from build123d import *

# Parameters (mm, degrees)
F0_R          = 4.5
F1_DEPTH      = 65
F2_W          = 24.1539999843
F2_H          = 28
F2_W_2        = 25
F2_W_3        = 30
F2_H_2        = 80
F3_DEPTH      = 45.001
F4_R          = 4.5
F5_DEPTH      = 45.001
F6_R          = 4.5
F7_DEPTH      = 6.5
F8_R          = 4.5
F9_DEPTH      = 14.5
F10_T4_DEPTH  = 132.8518303197
F10_S5_R      = 17.5
F10_T6_DEPTH  = 68
F10_T10_DEPTH = 132.8518303197
F10_S11_R     = 17.5
F10_T12_DEPTH = 68
F11_R         = 2


# Not quite as in the source:
# - a fillet or chamfer that OpenCascade refuses, or shapes differently, is made with other operations: its cross-section is extruded or revolved along the edge and cut away or added
# - a pattern or mirror of a feature is missing from the dataset's text; its kind, count and spacing are read off the source's solid


with BuildPart() as f1:
    # F0 (on Front) → F1 (new body, symmetric)
    with BuildSketch(Plane.XZ):
        with BuildLine():
            Line((80, 17.5), (0, 17.5))
            ThreePointArc((0, 17.5), (-17.2437155554, 2.9840029898), (-5.880605574, -16.4823687036))
            Line((-5.880605574, -16.4823687036), (25, -27.5))
            Line((25, -27.5), (55, -27.5))
            Line((55, -27.5), (85.880605574, -16.4823687036))
            ThreePointArc((85.880605574, -16.4823687036), (97.2437155554, 2.9840029898), (80, 17.5))
        make_face()
        Circle(F0_R, mode=Mode.SUBTRACT)
        with Locations((80, 0)):
            Circle(F0_R, mode=Mode.SUBTRACT)
    extrude(amount=F1_DEPTH, both=True)

    # F2 (on face) → F3 (cut, through all)
    with BuildSketch(Plane.XY.offset(17.5)):
        with Locations((-12.0769999921, 51)):
            Rectangle(F2_W, F2_H)
        with Locations((12.5, 51)):
            Rectangle(F2_W_2, F2_H)
        with Locations((-12.0769999921, -51)):
            Rectangle(F2_W, F2_H)
        with Locations((12.5, -51)):
            Rectangle(F2_W_2, F2_H)
        Polygon((55, 40), (55, 0), (55, -40), (80, -40), (80, 40), align=None)
        with Locations((95, 0)):
            Rectangle(F2_W_3, F2_H_2)
    extrude(amount=-F3_DEPTH, mode=Mode.SUBTRACT)

    # F4 (on face) → F5 (cut, through all)
    with BuildSketch(Plane(origin=(0, 0, -27.5), x_dir=(1, 0, 0), z_dir=(0, 0, -1))):
        with Locations((40, 50)):
            Circle(F4_R)
        with Locations((40, -50)):
            Circle(F4_R)
    extrude(amount=-F5_DEPTH, mode=Mode.SUBTRACT)

    # F6 (on face) → F7 (cut)
    with BuildSketch(Plane.XY.offset(17.5)):
        Polygon((35.9585481157, 43), (44.0414518843, 43), (48.0829037687, 50), (44.0414518843, 57), (35.9585481157, 57), (31.9170962313, 50), align=None)
        with Locations((40, 50)):
            Circle(F6_R, mode=Mode.SUBTRACT)
        Polygon((44.0414518843, -57), (48.0829037687, -50), (44.0414518843, -43), (35.9585481157, -43), (31.9170962313, -50), (35.9585481157, -57), align=None)
        with Locations((40, -50)):
            Circle(F6_R, mode=Mode.SUBTRACT)
    extrude(amount=-F7_DEPTH, mode=Mode.SUBTRACT)

    # F8 (on face) → F9 (join)
    with BuildSketch(Plane.XZ.offset(65)):
        with BuildLine():
            ThreePointArc((85.880605574, -16.4823687036), (94.3031569513, -10.0831394529), (97.5, 0))
            ThreePointArc((97.5, 0), (92.3743686708, 12.3743686708), (80, 17.5))
            ThreePointArc((80, 17.5), (62.7562844446, -2.9840029898), (85.880605574, -16.4823687036))
        make_face()
        with Locations((80, 0)):
            Circle(F8_R, mode=Mode.SUBTRACT)
    f9 = extrude(amount=F9_DEPTH)

    # F9_copies: F9 across plane
    add(f9.mirror(Plane.ZX))

    # F10: chamfer of 5 x 15 on 2 edges, made by hand


with BuildPart() as f10_tool2:
    # F10_s3 → F10_t4 (new body)
    with BuildSketch(Plane.YZ.offset(118.9259151598)):
        Polygon((-60, 17.5), (-65, 2.5), (-65, 17.5), align=None)
    extrude(amount=-F10_T4_DEPTH)

    # F10_s5 → F10_t6 (cut, symmetric)
    with BuildSketch(Plane.XZ.offset(62.5)):
        with Locations((80, 0)):
            Circle(F10_S5_R)
    extrude(amount=F10_T6_DEPTH, both=True, mode=Mode.SUBTRACT)


with BuildPart() as f1_1:
    add(f1.part)

    # F10_t1: cut F10_tool2
    add(f10_tool2.part, mode=Mode.SUBTRACT)


with BuildPart() as f10_tool8:
    # F10_s9 → F10_t10 (new body)
    with BuildSketch(Plane.YZ.offset(118.9259151598)):
        Polygon((60, 17.5), (65, 2.5), (65, 17.5), align=None)
    extrude(amount=-F10_T10_DEPTH)

    # F10_s11 → F10_t12 (cut, symmetric)
    with BuildSketch(Plane.XZ.offset(-62.5)):
        with Locations((80, 0)):
            Circle(F10_S11_R)
    extrude(amount=F10_T12_DEPTH, both=True, mode=Mode.SUBTRACT)


with BuildPart() as f1_2:
    add(f1_1.part)

    # F10_t7: cut F10_tool8
    add(f10_tool8.part, mode=Mode.SUBTRACT)

    # F11
    f11_edges = [f1_2.edges().sort_by_distance(p)[0] for p in [
        (55, -40, -5),
        (55, 40, -5),
    ]]
    fillet(f11_edges, radius=F11_R)


solid = f1_2.part
The model under review builds one solid part; all positions refer to its coordinate system, in mm. A direction names the side the tool comes from. Coordinates: 2 decimals unless noted, no trailing zeros. Write each loop counter-clockwise with the first axis right and the second up, starting at its lowest first coordinate (ties: lowest second). Pieces come first, ordered by that corner, then holes. Notation, with made-up numbers: (28.25, 32) -> (73.25, 32) arc R28 ccw to (73.25, 51) -> close; hole circle Ø1 at (49, 43.5). An arc over 180 degrees is marked (long way). Answer in a Markdown table with one row per item.
1. We need section D-D, the plane z = -21.5. State the section outline as (x, y) points, and give its area (3 significant figures).
Answers below:
| item | result |
|---|---|
| outline | (8.18, -37) -> (25, -37) -> (25, -65) -> (71.82, -65) -> (71.82, -40) -> (57, -40) arc R2 cw to (55, -38) -> (55, 38) arc R2 cw to (57, 40) -> (71.82, 40) -> (71.82, 65) -> (25, 65) -> (25, 37) -> (8.18, 37) -> close; hole circle Ø9 at (40, -50); hole circle Ø9 at (40, 50) |
| area | 5,860 mm^2 |
2. For faces 1 (the flat face through (46.774, 62.465, 10.105)), 2 (the cylindrical face through (95.577, 63.862, 7.976)), 3 (the flat face through (46.034, 46.451, 14.296)), 4 (the flat face through (73, 40, 1)), 5 (the flat face through (9, -37, 0)), list the 3-axis set-ups (+Z, -Z, +X, -X, +Y, -Y) from which the entire face can be reached by the end or side of a thin tool; tool diameter is ignored.
Answers below:
| item | result |
|---|---|
| face 1 | +Z, -X, +Y |
| face 2 | +Y |
| face 3 | +Z |
| face 4 | +Z, -Z, +X |
| face 5 | +Z, -Z, -X, -Y |
3. Clearance check with flat-ended pins moving along their axes: pin 1 Ø12.5 at (x, z) = (-5, -2.5) entering from -Y; pin 2 Ø12 at (x, z) = (29.5, -5.5) entering from +Y; pin 3 Ø7 at (x, z) = (80, 0) entering from +Y; pin 4 Ø4 at (y, z) = (49.5, 4.5) entering from +X. State where each tip first meets the part, or that it passes through.
Answers below:
| item | result |
|---|---|
| pin 1 | stops at y = -37 |
| pin 2 | stops at y = 65 |
| pin 3 | passes through |
| pin 4 | stops at x = 97.32 |
4. We need section A-A, the plane x = 40. State the section outline as (y, z) points.
Answers below:
| item | result |
|---|---|
| outline | (-65, -27.5) -> (-54.5, -27.5) -> (-54.5, 11) -> (-57, 11) -> (-57, 17.5) -> (-60, 17.5) -> (-65, 2.5) -> close; (-45.5, -27.5) -> (45.5, -27.5) -> (45.5, 11) -> (43, 11) -> (43, 17.5) -> (-43, 17.5) -> (-43, 11) -> (-45.5, 11) -> close; (54.5, -27.5) -> (65, -27.5) -> (65, 2.5) -> (60, 17.5) -> (57, 17.5) -> (57, 11) -> (54.5, 11) -> close |
5. Draft analysis for pull direction Y (two halves, no side actions). For faces 6 (the flat face through (84, 79.5, -4)), 7 (the flat face through (40, -1, -27.5)), 8 (the flat face through (84, -79.5, -4)), 9 (the cylindrical face through (42.08, -46.01, -8.52)), state which applies: +Y half, -Y half, draft (parallel to the pull), parting line (faces both ways), or undercut.
Answers below:
| item | result |
|---|---|
| face 6 | +Y half |
| face 7 | draft |
| face 8 | -Y half |
| face 9 | undercut |
6. We need section C-C, the plane x = 88. State the section outline as (y, z) points, and give its area (3 significant figures).
Answers below:
| item | result |
|---|---|
| outline | (-79.5, -15.56) -> (-40, -15.56) -> (-40, 15.56) -> (-79.5, 15.56) -> close; (40, -15.56) -> (79.5, -15.56) -> (79.5, 15.56) -> (40, 15.56) -> close |
| area | 2,460 mm^2 |
7. We need section B-B, the plane z = -6.5. State the section outline as (x, y) points.
Answers below:
| item | result |
|---|---|
| outline | (-16.25, -37) -> (25, -37) -> (25, -65) -> (63.75, -65) -> (63.75, -79.5) -> (96.25, -79.5) -> (96.25, -40) -> (57, -40) arc R2 cw to (55, -38) -> (55, 38) arc R2 cw to (57, 40) -> (96.25, 40) -> (96.25, 79.5) -> (63.75, 79.5) -> (63.75, 65) -> (25, 65) -> (25, 37) -> (-16.25, 37) -> close; hole circle Ø9 at (40, -50); hole circle Ø9 at (40, 50) |
8. Wall thickness on probe 1 along Y at (x, z) = (40, -13.5); probe 2 along X at (y, z) = (50, 0.5); probe 3 along Y at (x, z) = (87, 15): over which ranges is each line inside the solid? List them lowest first. Write a range as [from, to].
Answers below:
| item | result |
|---|---|
| probe 1 | y = [-65, -54.5], [-45.5, 45.5], [54.5, 65] |
| probe 2 | x = [25, 35.5], [44.5, 75.53], [84.47, 97.49] |
| probe 3 | y = [-79.5, -40], [40, 79.5] |
